```python
from build123d import *

# Parameters (mm, degrees)
SZKIC1_R                    = 13
DODANIE_WYCI_GNI_CIE1_DEPTH = 6
ZAOKR_GLENIE1_R             = 0.2


with BuildPart() as part:
    # Szkic1 → Dodanie-wyciągnięcie1 (new body, symmetric)
    with BuildSketch(Plane(origin=(0, 0, 0), x_dir=(1, 0, 0), z_dir=(0, 1, 0))):
        Circle(SZKIC1_R)
    extrude(amount=DODANIE_WYCI_GNI_CIE1_DEPTH, both=True)

    # Szkic3 → Wycięcie-obrót1 (revolve, cut)
    with BuildSketch(Plane.XY):
        with BuildLine():
            Line((0, -11.1), (0, 11.1))
            ThreePointArc((0, 11.1), (11.1, 0), (0, -11.1))
        make_face()
    revolve(axis=Axis((0, -11.1, 0), (0, 1, 0)), mode=Mode.SUBTRACT)

    # Zaokrąglenie1
    zaokr_glenie1_edges = [part.edges().sort_by_distance(p)[0] for p in [
        (-13, -6, 0),
        (-13, 6, 0),
    ]]
    fillet(zaokr_glenie1_edges, radius=ZAOKR_GLENIE1_R)


solid = part.part
```
The model under review builds one solid part; all positions refer to its coordinate system, in mm. Coordinates: 2 decimals unless noted, no trailing zeros. Loops run counter-clockwise (first coordinate to the right, second up) from the corner with the lowest first, then second, coordinate; pieces in that order, holes last. Notation, with made-up numbers: (4, 48) -> (28, 48) arc R34 ccw to (28, 86) -> close; hole circle Ø5 at (43.5, -2.75). An arc over 180 degrees is marked (long way). Answer as CSV lines item,"result".
Item 1: Take a section at B-B, the plane y = 0. State the section outline as (x, z) points, and give its area (3 significant figures).
Results below:
outline,"circle Ø26 at (0, 0); hole circle Ø22.2 at (0, 0)"
area,"144 mm2"
Item 2: For L1, parallel to X at y = -1, z = 7.5; L2, parallel to Z at x = 4.25, y = -1; L3, parallel to Z at x = 2.75, y = 4.5, list the stretches that pass through material, from the lowest coordinate up.
Results below:
L1,"x = -10.62 to -8.12, 8.12 to 10.62"
L2,"z = -12.29 to -10.21, 10.21 to 12.29"
L3,"z = -12.71 to -9.77, 9.77 to 12.71"
Item 3: Insertion check: pin 1 (2 mm diameter, centred on x = -6.5, y = -2.5, fed in from -Z); pin 2 (4 mm diameter, centred on y = -0.5, z = -8.5, fed in from +X); pin 3 (6 mm diameter, centred on y = -3, z = -8.5, fed in from +X). Each pin has a flat end and moves straight along its axis. Give the tip position at first contact, or say it passes through.
Results below:
pin 1,"stops at z = -11.78"
pin 2,"stops at x = 11.26"
pin 3,"stops at x = 11.78"
Item 4: Take a section at D-D, the plane y = 3.25. State the section outline as (x, z) points, and give its area (3 significant figures).
Results below:
outline,"circle Ø26 at (0, 0); hole circle Ø21.23 at (0, 0)"
area,"177 mm2"
Item 5: Take a section at C-C, the plane x = 0. State the section outline as (y, z) points.
Results below:
outline,"(-6, -12.8) arc R0.2 ccw to (-5.8, -13) -> (5.8, -13) arc R0.2 ccw to (6, -12.8) -> (6, -9.34) arc R11.1 cw to (-6, -9.34) -> close; (-6, 9.34) arc R11.1 cw to (6, 9.34) -> (6, 12.8) arc R0.2 ccw to (5.8, 13) -> (-5.8, 13) arc R0.2 ccw to (-6, 12.8) -> close"
Item 6: Take a section at A-A, the plane z = 0. State the section outline as (x, y) points, and give its area (3 significant figures).
Results below:
outline,"(-13, -5.8) arc R0.2 ccw to (-12.8, -6) -> (-9.34, -6) arc R11.1 cw to (-9.34, 6) -> (-12.8, 6) arc R0.2 ccw to (-13, 5.8) -> close; (9.34, -6) -> (12.8, -6) arc R0.2 ccw to (13, -5.8) -> (13, 5.8) arc R0.2 ccw to (12.8, 6) -> (9.34, 6) arc R11.1 cw to start"
area,"59.2 mm2"
